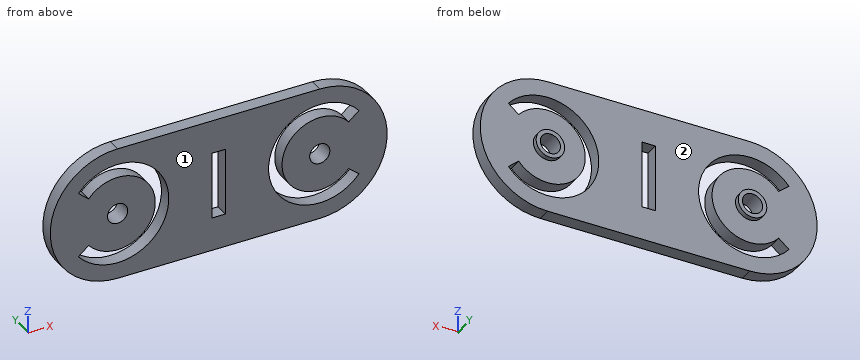
from build123d import *

# Parameters (mm, degrees)
BOSS_EXTRUDE1_DEPTH = 4.000000128
SKETCH2_R           = 2.999994
SKETCH2_W           = 3.999992
SKETCH2_H           = 20.0000108
CUT_EXTRUDE1_DEPTH  = 54.999999958
BOSS_EXTRUDE2_START = 1.499997
SKETCH3_R           = 4.2333418
SKETCH3_R_2         = 2.999994
BOSS_EXTRUDE2_DEPTH = 1.499997


with BuildPart() as part:
    # Sketch1 → Boss-Extrude1 (new body)
    with BuildSketch(Plane(origin=(0, 0, 0), x_dir=(1, 0, 0), z_dir=(0, 1, 0))):
        with BuildLine():
            Line((-29.999999944, 20), (29.999999944, 20))
            ThreePointArc((29.999999944, 20), (49.999999944, 0), (29.999999944, -20))
            Line((29.999999944, -20), (-29.999999944, -20))
            ThreePointArc((-29.999999944, -20), (-49.999999944, 0), (-29.999999944, 20))
        make_face()
    extrude(amount=BOSS_EXTRUDE1_DEPTH)

    # Sketch2 → Cut-Extrude1 (cut, through all)
    with BuildSketch(Plane(origin=(0, 4.000000128, 0), x_dir=(1, 0, 0), z_dir=(0, 1, 0))):
        with Locations(Location((-29.999999944, 0, 0), (0, 0, 270))):
            Circle(SKETCH2_R)
        with Locations(Location((29.999999944, 0, 0), (0, 0, 90))):
            Circle(SKETCH2_R)
        Rectangle(SKETCH2_W, SKETCH2_H)
        with BuildLine():
            Line((-41.640032544, 9.7671636), (-38.575878144, 7.1959978))
            ThreePointArc((-38.575878144, 7.1959978), (-18.804997879, 0), (-38.575878144, -7.1959978))
            Line((-38.575878144, -7.1959978), (-41.640032544, -9.7671636))
            ThreePointArc((-41.640032544, -9.7671636), (-14.805005909, 0), (-41.640032544, 9.7671636))
        make_face()
        with BuildLine():
            Line((41.640032544, -9.7671636), (38.575878144, -7.1959978))
            ThreePointArc((38.575878144, -7.1959978), (18.804997879, 0), (38.575878144, 7.1959978))
            Line((38.575878144, 7.1959978), (41.640032544, 9.7671636))
            ThreePointArc((41.640032544, 9.7671636), (14.805005909, 0), (41.640032544, -9.7671636))
        make_face()
    extrude(amount=-CUT_EXTRUDE1_DEPTH, mode=Mode.SUBTRACT)

    # Sketch3 → Boss-Extrude2 (add)
    # profile 1 of 2: a face of its own
    with BuildSketch(Plane(origin=(0, 4.000000128, 0), x_dir=(1, 0, 0), z_dir=(0, 1, 0)).offset(BOSS_EXTRUDE2_START)):
        with Locations(Location((-29.999999944, 0, 0), (0, 0, 270))):
            Circle(SKETCH3_R)
        with Locations(Location((-29.999999944, 0, 0), (0, 0, 270))):
            Circle(SKETCH3_R_2, mode=Mode.SUBTRACT)
    # profile 2 of 2: a face of its own
    with BuildSketch(Plane(origin=(0, 4.000000128, 0), x_dir=(1, 0, 0), z_dir=(0, 1, 0)).offset(BOSS_EXTRUDE2_START)):
        with Locations(Location((29.999999944, 0, 0), (0, 0, 90))):
            Circle(SKETCH3_R)
        with Locations(Location((29.999999944, 0, 0), (0, 0, 90))):
            Circle(SKETCH3_R_2, mode=Mode.SUBTRACT)
    extrude(amount=-BOSS_EXTRUDE2_DEPTH)


solid = part.part
Model file for the job. Use its own axes, mm. Face numbers are marked on the shaded views. Give positions to 0.01 mm unless a question says otherwise; leave off trailing zeros. Write each loop counter-clockwise with the first axis right and the second up, starting at its lowest first coordinate (ties: lowest second). Pieces come first, ordered by that corner, then holes. Notation, with made-up numbers: M 19,-25.5 L 70,-25.5 A30 cw 70,9.5 Z; hole C -33.75,25 d2. An arc over 180 degrees is marked long. One line per item, written item: value. Start each with the question number.
Q1. Two-plate mould, pull along X, no slides. Class the marked faces 1 and 2: +X half, -X half, draft (parallel to the pull), parting line (faces both ways), or undercut.
Q2. Saw through at A-A, the plane z = 0. State how many separate pieces and enclosed holes the cut face has, plus the area to 3 significant figures.
Q3. Probe probe 1 along Z at (x, y) = (30, 2.95) (3 decimals); probe 2 along X at (y, z) = (1.7, 0) (3 decimals); probe 3 along X at (y, z) = (3.4, 14). List the from-to ranges inside material, lowest first. Write a range as [from, to].
Q4. Saw through at D-D, the plane z = 13. Write the cut outline in (x, y).
Q5. Saw through at C-C, the plane x = 31. Write the cut outline in (y, z), plus the area to 3 significant figures.
Q6. Drop flat-ended pins along their axis: pin 1 Ø2 at (y, z) = (1.5, -4) entering from -X; pin 2 Ø2 at (x, y) = (-36.5, 2) entering from -Z; pin 3 Ø3 at (y, z) = (1, -1.5) entering from +X; pin 4 Ø1 at (x, z) = (-28, 5.5) entering from -Y. Give the stop position or say it passes through.
Q7. Saw through at B-B, the plane y = 2. Write the cut outline in (x, z) (3 decimals).
Output values:
1. face 1: draft
1. face 2: undercut
2. separate pieces: 6
2. enclosed holes: 0
2. area: 311 mm²
3. probe 1: z = [-20, -15.195], [-11.195, -3], [3, 11.195], [15.195, 20]
3. probe 2: x = [-50, -33], [-27, -18.805], [-14.805, -2], [2, 14.805], [18.805, 27], [33, 50]
3. probe 3: x = [-44.28, -35.91], [-24.09, 24.09], [35.91, 44.28]
4. outline: M -45.2,0 L -37.87,0 L -37.87,4 L -45.2,4 Z; M -22.13,0 L 22.13,0 L 22.13,4 L -22.13,4 Z; M 37.87,0 L 45.2,0 L 45.2,4 L 37.87,4 Z
5. outline: M 0,-19.97 L 4,-19.97 L 4,-15.16 L 0,-15.16 Z; M 0,-11.15 L 4,-11.15 L 4,-4.11 L 5.5,-4.11 L 5.5,-2.83 L 0,-2.83 Z; M 0,2.83 L 5.5,2.83 L 5.5,4.11 L 4,4.11 L 4,11.15 L 0,11.15 Z; M 0,15.16 L 4,15.16 L 4,19.97 L 0,19.97 Z
5. area: 109 mm²
6. pin 1: stops at x = -49.77
6. pin 2: stops at z = -19.23
6. pin 3: stops at x = 50
6. pin 4: stops at y = 0
7. outline: M -30,-20 L 30,-20 A20 ccw 30,20 L -30,20 A20 ccw Z; hole M -41.64,-9.767 A15.195 ccw long -41.64,9.767 L -38.576,7.196 A11.195 cw long -38.576,-7.196 Z; hole C -30,0 d6; hole M -2,-10 L 2,-10 L 2,10 L -2,10 Z; hole C 30,0 d6; hole M 38.576,-7.196 A11.195 cw long 38.576,7.196 L 41.64,9.767 A15.195 ccw long 41.64,-9.767 Z
